Could you check a few things on this model? Use its own coordinates, in mm. Face numbers are marked on the shaded views. A direction names the side the tool comes from. Give positions to 0.01 mm unless a question says otherwise; leave off trailing zeros. Loops run counter-clockwise (first coordinate to the right, second up) from the corner with the lowest first, then second, coordinate; pieces in that order, holes last. Notation, with made-up numbers: (47, 22.5) - (99, 22.5) arc R34 ccw to (99, 56.5) - close; hole circle Ø6 at (-34.75, 45). An arc over 180 degrees is marked (long way). One line per item, written item: value. Start each with the question number.
Q1. I want a section at C-C (x = -12.5). Please give me the cut outline in (y, z).
Q2. I want a section at A-A (x = -25). Please give me the cut outline in (y, z), then the cut area to 3 significant figures.
Q3. I'm going to push flat-ended pins straight in: P1, Ø5, axis at x = -6.5, y = 1, coming from the +Z side; P2, Ø5, axis at x = 3, y = -14, coming from the +Z side; P3, Ø1.1, axis at x = -56.5, y = 0.5, coming from the +Z side. Where does each tip first touch, or does it pass through?
Q4. For the marked faces 1 and 2, which set-ups out of +Z, -Z, +X, -X, +Y, -Y let a thin tool reach every point of the face, with its end or its side?
Q5. I want a section at B-B (y = 0). Count the separate pieces of the cut face and the enclosed holes in it, then the cut area to 3 significant figures.
Q6. If I drill on line 1 (X direction, y = 13, z = 0.3); line 2 (Y direction, x = 48, z = 4.85); line 3 (Y direction, x = 3, z = 2.5), over which ranges is the centre line in solid material (lowest first)? Write a range as from..to.
Q7. If we mould it in two halves opening along Y, with no side actions, what happens to the marked faces 3, 4 and 5? For each: released by +Y, released by -Y, zero draft, split by the parting line, or undercut.
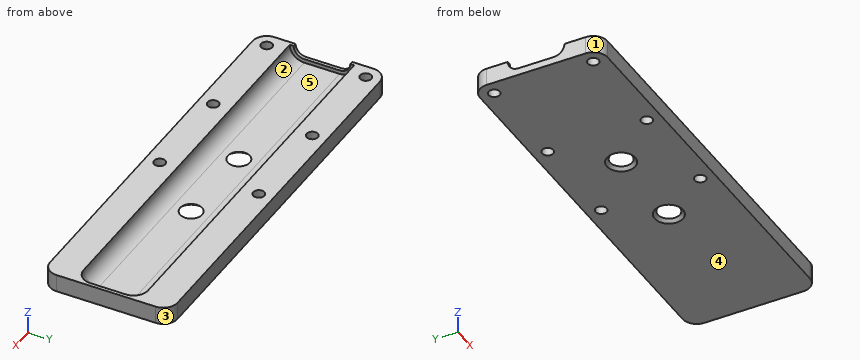
Solid Edge part; units mm, degrees
sketch "Sketch1" plane through (0, 0, 0) normal (0, 0, 1) x (1, 0, 0)
  line L0 (57, -18) -> (57, 18)
  line L1 (57, 18) -> (-57, 18)
  line L2 (-57, 18) -> (-57, -18)
  line L3 (-57, -18) -> (57, -18)
extrude "Protrusion1" add sketch "Sketch1" along normal blind 5
sketch "Sketch2" plane through (-57, 0, 2.5) normal (-1, 0, 0) x (0, -1, 0)
  line L0 (-5, -0.5) -> (5, -0.5)
  line L1 (-8, 2.5) -> (8, 2.5)
  arc A0 (8, 2.5) -> (5, -0.5) centre (5, 2.5) cw
  arc A1 (-5, -0.5) -> (-8, 2.5) centre (-5, 2.5) cw
extrude "VaciadoExtruido_2" cut sketch "Sketch2" against normal blind 1
sketch "Sketch3" plane through (-56, 0, 2.5) normal (-1, 0, 0) x (0, -1, 0)
  line L0 (-5, -1.6) -> (5, -1.6)
  line L1 (-9.1, 2.5) -> (9.1, 2.5)
  arc A0 (9.1, 2.5) -> (5, -1.6) centre (5, 2.5) cw
  arc A1 (-5, -1.6) -> (-9.1, 2.5) centre (-5, 2.5) cw
extrude "VaciadoExtruido_3" cut sketch "Sketch3" against normal blind 112
fillet "Redondeo_3" radius 4.1 3 edges at (56, 7.8991, 2.1009) (56, -7.8991, 2.1009) (56, 0, 0.9)
sketch "Sketch4" plane through (0, 0, 5) normal (0, 0, 1) x (1, 0, 0)
  circle A0 centre (-53, 14) radius 1.6
extrude "Cutout1" cut sketch "Sketch4" against normal through all
pattern_linear "Pattern1" count 3 spacing 28 along (1, 0, 0) count 2 spacing 28 along (0, -1, 0) of "Cutout1"
fillet "Redondeo_4" radius 4 4 edges at (-57, 18, 2.5) (-57, -18, 2.5) (57, 18, 2.5) (57, -18, 2.5)
sketch "Sketch5" plane through (0, 0, 0) normal (0, 0, -1) x (1, 0, 0)
  circle A0 centre (12.5, 0) radius 3
  circle A1 centre (-12.5, 0) radius 3
extrude "Cutout2" cut sketch "Sketch5" against normal through all
chamfer "Chaflán_1" distance 1 angle 45 2 edges at (-15.5, 0, 0) (9.5, 0, 0)
Worked answers:
1. outline: (-18, 0) - (-4, 0) - (-3.1, 0.9) - (-5, 0.9) arc R4.1 cw to (-9.1, 5) - (-18, 5) - close; (3.1, 0.9) - (4, 0) - (18, 0) - (18, 5) - (9.1, 5) arc R4.1 cw to (5, 0.9) - close
2. outline: (-18, 0) - (-15.6, 0) - (-15.6, 5) - (-18, 5) - close; (-12.4, 0) - (12.4, 0) - (12.4, 5) - (9.1, 5) arc R4.1 cw to (5, 0.9) - (-5, 0.9) arc R4.1 cw to (-9.1, 5) - (-12.4, 5) - close; (15.6, 0) - (18, 0) - (18, 5) - (15.6, 5) - close
2. area: 80.6 mm²
3. P1: stops at z = 0.9
3. P2: stops at z = 5
3. P3: stops at z = 2
4. face 1: +Z, -Z, -X, -Y
4. face 2: +Z
5. separate pieces: 3
5. enclosed holes: 0
5. area: 98.6 mm²
6. line 1: x = -57..-54.25, -51.75..-26.25, -23.75..1.75, 4.25..57
6. line 2: y = -18..-9.1, 9.1..18
6. line 3: y = -18..-15.6, -12.4..-8.25, 8.25..12.4, 15.6..18
7. face 3: released by +Y
7. face 4: zero draft
7. face 5: undercut
